```python
from build123d import *

# Parameters (mm, degrees)
F0_R          = 38.1
F1_DEPTH      = 2.54
F2_R          = 12.7
F3_DEPTH      = 29.21
F4_R          = 10.6934
F5_DEPTH      = 6.35
F6_R          = 38.1
F7_DEPTH      = 2.54
F8_R          = 3.1115
F9_DEPTH      = 25.4
F9_DEPTH_BACK = 25.4
F10_SIZE      = 3.81


with BuildPart() as f1:
    # F0 (on Front) → F1 (new body)
    with BuildSketch(Plane.XZ):
        Circle(F0_R)
    extrude(amount=-F1_DEPTH)

    # F2 (on Front) → F3 (join)
    with BuildSketch(Plane.XZ):
        Circle(F2_R)
    extrude(amount=-F3_DEPTH)

    # F4 (on Front) → F5 (cut)
    with BuildSketch(Plane.XZ):
        Circle(F4_R)
    extrude(amount=-F5_DEPTH, mode=Mode.SUBTRACT)

    # F6 (on face) → F7 (join)
    with BuildSketch(Plane(origin=(0, 29.21, 0), x_dir=(-1, 0, 0), z_dir=(0, 1, 0))):
        Circle(F6_R)
    extrude(amount=F7_DEPTH)

    # F8 (on Right) → F9 (cut, two sides)
    with BuildSketch(Plane.YZ) as f9_sk:
        with Locations((14.287057, 0)):
            Circle(F8_R)
    extrude(amount=F9_DEPTH, mode=Mode.SUBTRACT)
    extrude(f9_sk.sketch, amount=-F9_DEPTH_BACK, mode=Mode.SUBTRACT)

    # F10
    f10_edges = [f1.edges().sort_by_distance(p)[0] for p in [
        (-12.7, 2.54, 0),
    ]]
    chamfer(f10_edges, length=F10_SIZE)


solid = f1.part
```
Could you check a few things on this model? Use its own coordinates, in mm. A direction names the side the tool comes from. Coordinates: 2 decimals unless noted, no trailing zeros. Write each loop counter-clockwise with the first axis right and the second up, starting at its lowest first coordinate (ties: lowest second). Pieces come first, ordered by that corner, then holes. Notation, with made-up numbers: (60, -10) -> (66, -10) arc R20 ccw to (66, 28) -> close; hole circle Ø9 at (-30, 29). An arc over 180 degrees is marked (long way). Return JSON: item names as keys, results as strings.
(1) I'm going to push flat-ended pins straight in: pin 1 (5 mm diameter, centred on x = 17, y = 17.5, fed in from -Z); pin 2 (7 mm diameter, centred on y = 14.29, z = 0, fed in from -X); pin 3 (12 mm diameter, centred on x = -17, y = 27.5, fed in from +Z); pin 4 (12 mm diameter, centred on x = -30, z = -8, fed in from -Y). Where does each tip first touch, or does it pass through?
Numbers:
{"pin 1": "passes through", "pin 2": "stops at x = -12.7", "pin 3": "stops at z = 36.4", "pin 4": "stops at y = 0"}
(2) Imagine slicing it at B-B, the plane x = 32.5. Please give me the cut outline in (y, z).
Numbers:
{"outline": "(0, -19.88) -> (2.54, -19.88) -> (2.54, 19.88) -> (0, 19.88) -> close; (29.21, -19.88) -> (31.75, -19.88) -> (31.75, 19.88) -> (29.21, 19.88) -> close"}
(3) We'd pull the mould along X, two halves only. Please class faces 3 (the flat face through (0, 6.35, 0)), 4 (the conical face through (12.34, 6.11, 3.89)), 5 (the flat face through (1, 31.75, 1)), 6 (the cylindrical face through (-8.486, 3.131, -6.507)): +X half, -X half, draft (parallel to the pull), parting line (faces both ways), or undercut.
Numbers:
{"face 3": "undercut", "face 4": "parting line", "face 5": "draft", "face 6": "undercut"}
(4) I need wall thicknesses on L1, parallel to Y at x = -16.5, z = -28; L2, parallel to Y at x = 6.75, z = 0; L3, parallel to Y at x = 5, z = -7. Which ranges of each line are inside material? Lowest first, please.
Numbers:
{"L1": "y = 0 to 2.54, 29.21 to 31.75", "L2": "y = 6.35 to 11.18, 17.4 to 31.75", "L3": "y = 6.35 to 31.75"}
(5) Which directions (+Z, -Z, +X, -X, +Y, -Y) give clear straight access to the entire face, cutting with the end or side of a thin tool? Please do faces 1 (the cylindrical face through (-30.235, 1.252, -23.183)), 2 (the flat face through (16, 2.54, -8)).
Numbers:
{"face 1": "+Y, -Y", "face 2": "none"}
(6) Imagine slicing it at C-C, the plane y = 3.5. Please give me the cut outline in (x, z), then the cut area to 3 significant figures.
Numbers:
{"outline": "circle Ø31.1 at (0, 0); hole circle Ø21.39 at (0, 0)", "area": "400 mm2"}
(7) Imagine slicing it at D-D, the plane x = -31. Please give me the cut outline in (y, z), then the cut area to 3 significant figures.
Numbers:
{"outline": "(0, -22.15) -> (2.54, -22.15) -> (2.54, 22.15) -> (0, 22.15) -> close; (29.21, -22.15) -> (31.75, -22.15) -> (31.75, 22.15) -> (29.21, 22.15) -> close", "area": "225 mm2"}
(8) Imagine slicing it at A-A, the plane z = 0. Please give me the cut outline in (x, y), then the cut area to 3 significant figures.
Numbers:
{"outline": "(-38.1, 0) -> (-10.69, 0) -> (-10.69, 6.35) -> (10.69, 6.35) -> (10.69, 0) -> (38.1, 0) -> (38.1, 2.54) -> (16.51, 2.54) -> (12.7, 6.35) -> (12.7, 11.18) -> (-12.7, 11.18) -> (-12.7, 6.35) -> (-16.51, 2.54) -> (-38.1, 2.54) -> close; (-38.1, 29.21) -> (-12.7, 29.21) -> (-12.7, 17.4) -> (12.7, 17.4) -> (12.7, 29.21) -> (38.1, 29.21) -> (38.1, 31.75) -> (-38.1, 31.75) -> close", "area": "785 mm2"}
